Read the model definition and answer for the solid it produces. Units are mm, in the model's axes. Face numbers are marked on the shaded views. A direction names the side the tool comes from. Give positions to 0.01 mm unless a question says otherwise; leave off trailing zeros. Write each loop counter-clockwise with the first axis right and the second up, starting at its lowest first coordinate (ties: lowest second). Pieces come first, ordered by that corner, then holes. Notation, with made-up numbers: (84.5, 41) -> (98.5, 41) arc R18 ccw to (98.5, 63) -> close; hole circle Ø9 at (36.25, -1). An arc over 180 degrees is marked (long way). Answer as CSV lines item,"result". Start each with the question number.
1. A tool of negligible diameter and unlimited length cuts with its end or side. For the marked faces 1 and 2, from which of +Z, -Z, +X, -X, +Y, -Y can it reach the whole face along a straight path? Write none if from no direction.
2. Find the intervals of material crossed by line 1 (Z direction, x = -1.2, y = 1.5); line 2 (Z direction, x = 0, y = -0.8); line 3 (X direction, y = -0.55, z = -2), in increasing order.
3. The part is cut by section C-C, the plane z = -1.25. Determine the outline of the cut face in (x, y), and give its area (3 significant figures).
4. The part is cut by section B-B, the plane y = 0. Determine the outline of the cut face in (x, z).
5. The part is cut by section A-A, the plane z = -4. Determine the outline of the cut face in (x, y).
6. Given pin 1 (1.5 mm diameter, centred on y = 1, z = -2.5, fed in from +X); pin 2 (1 mm diameter, centred on x = -1.5, z = 0.5, fed in from -Y); pin 3 (0.8 mm diameter, centred on x = 0, y = 0, fed in from -Z), each flat-ended and moving along its own axis, determine where each tip first touches the part or whether it passes through.
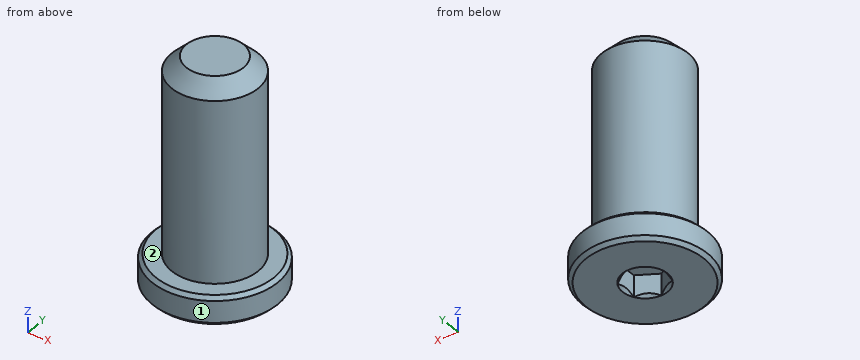
from build123d import *

# Parameters (mm, degrees)
EXTRUDE1_START     = -3.38455
SKETCH1_R          = 1.7526
EXTRUDE1_DEPTH     = 7.9375
EXTRUDE2_START     = -4.55295
SKETCH6_R          = 2.54
EXTRUDE2_DEPTH     = 1.1684
CUT_EXTRUDE1_DEPTH = 0.8763
SKETCH8_R          = 0.916543552
CUT_EXTRUDE2_DEPTH = 0.8763
CUT_EXTRUDE2_TAPER = 45
CHAMFER1_SIZE      = 0.14605
CHAMFER2_SIZE      = 0.5953125


with BuildPart() as part:
    # Sketch1 → Extrude1 (new body)
    with BuildSketch(Plane.XY.offset(EXTRUDE1_START)):
        Circle(SKETCH1_R)
    extrude(amount=EXTRUDE1_DEPTH)

    # Sketch6 → Extrude2 (add)
    with BuildSketch(Plane.XY.offset(EXTRUDE2_START)):
        Circle(SKETCH6_R)
    extrude(amount=EXTRUDE2_DEPTH)

    # Sketch7 → Cut-Extrude1 (cut)
    with BuildSketch(Plane.XY.offset(-4.55295)):
        Polygon((0, 0.916543552), (-0.79375, 0.458271776), (-0.79375, -0.458271776), (0, -0.916543552), (0.79375, -0.458271776), (0.79375, 0.458271776), align=None)
    extrude(amount=CUT_EXTRUDE1_DEPTH, mode=Mode.SUBTRACT)

    # Sketch8 → Cut-Extrude2 (cut)
    with BuildSketch(Plane.XY.offset(-4.55295)):
        Circle(SKETCH8_R)
    extrude(amount=CUT_EXTRUDE2_DEPTH, taper=CUT_EXTRUDE2_TAPER, mode=Mode.SUBTRACT)

    # Chamfer1
    chamfer1_edges = [part.edges().sort_by_distance(p)[0] for p in [
        (-2.54, 0, -3.38455),
        (-2.54, 0, -4.55295),
    ]]
    chamfer(chamfer1_edges, length=CHAMFER1_SIZE)

    # Chamfer2
    chamfer2_edges = [part.edges().sort_by_distance(p)[0] for p in [
        (-1.7526, 0, 4.55295),
    ]]
    chamfer(chamfer2_edges, length=CHAMFER2_SIZE)


solid = part.part
Results found:
1,face 1,"+Z, -Z"
1,face 2,"+Z"
2,line 1,"z = -4.55 to -3.38"
2,line 2,"z = -3.68 to 4.55"
2,line 3,"x = -1.66 to 1.66"
3,outline,"circle Ø3.51 at (0, 0)"
3,area,"9.65 mm²"
4,outline,"(-2.54, -4.41) -> (-2.39, -4.55) -> (-0.92, -4.55) -> (-0.79, -4.43) -> (-0.79, -3.68) -> (0.79, -3.68) -> (0.79, -4.43) -> (0.92, -4.55) -> (2.39, -4.55) -> (2.54, -4.41) -> (2.54, -3.53) -> (2.39, -3.38) -> (1.75, -3.38) -> (1.75, 3.96) -> (1.16, 4.55) -> (-1.16, 4.55) -> (-1.75, 3.96) -> (-1.75, -3.38) -> (-2.39, -3.38) -> (-2.54, -3.53) -> close"
5,outline,"circle Ø5.08 at (0, 0); hole (-0.79, -0.46) -> (0, -0.92) -> (0.79, -0.46) -> (0.79, 0.46) -> (0, 0.92) -> (-0.79, 0.46) -> close"
6,pin 1,"stops at x = 1.73"
6,pin 2,"stops at y = -1.44"
6,pin 3,"stops at z = -3.68"
